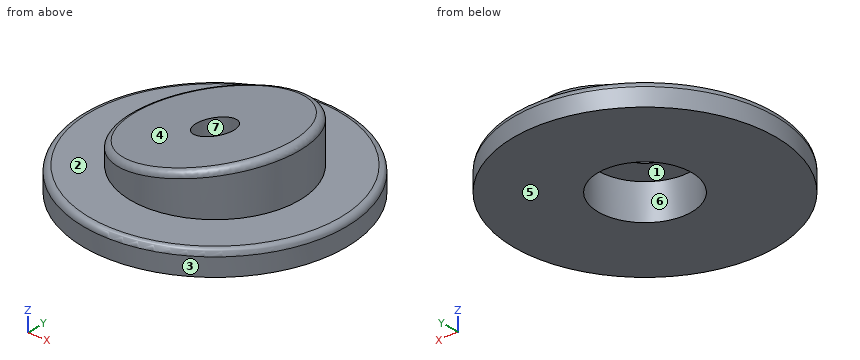
```python
from build123d import *

# Parameters (mm, degrees)
F0_R          = 11.1125
F0_R_2        = 7.14375
F1_DEPTH      = 2.032
F0_R_3        = 1.5875
F2_DEPTH      = 6.35
F4_DEPTH      = 11.1135
F4_DEPTH_BACK = 11.1135
F5_R          = 3.96875
F5_R_2        = 1.5875
F6_DEPTH      = 3.048
F7_R          = 0.508


with BuildPart() as f1:
    # F0 (on Top) → F1 (new body)
    with BuildSketch(Plane.XY):
        Circle(F0_R)
        Circle(F0_R_2, mode=Mode.SUBTRACT)
    extrude(amount=F1_DEPTH)

    # F0 (on Top) → F2 (join)
    with BuildSketch(Plane.XY):
        Circle(F0_R_2)
        Circle(F0_R_3, mode=Mode.SUBTRACT)
    extrude(amount=F2_DEPTH)

    # F3 (on Front) → F4 (cut, two sides)
    with BuildSketch(Plane.XZ) as f4_sk:
        Polygon((7.14375, 6.35), (-7.14375, 6.35), (-7.14375, 3.3864264842), align=None)
    extrude(amount=-F4_DEPTH, mode=Mode.SUBTRACT)
    extrude(f4_sk.sketch, amount=F4_DEPTH_BACK, mode=Mode.SUBTRACT)

    # F5 (on face) → F6 (cut)
    with BuildSketch(Plane(origin=(0, 0, 0), x_dir=(1, 0, 0), z_dir=(0, 0, -1))):
        Circle(F5_R)
        Circle(F5_R_2, mode=Mode.SUBTRACT)
    extrude(amount=-F6_DEPTH, mode=Mode.SUBTRACT)

    # F7
    f7_edges = [f1.edges().sort_by_distance(p)[0] for p in [
        (0, -7.14375, 4.868213),
        (0, 7.14375, 4.868213),
        (-11.1125, 0, 2.032),
    ]]
    fillet(f7_edges, radius=F7_R)


solid = f1.part
```
Source: CAD feature listing. Evaluate the final solid. Frame: model axes, mm. Face numbers are marked on the shaded views. A direction names the side the tool comes from. Coordinates: 2 decimals unless noted, no trailing zeros. Answer as a JSON object with one key per item and string values.
Q1. Draft query along X for the marked faces 4, 5, 6 and 7. Return one class per face: released by +X, released by -X, zero draft, split by the parting line, or undercut.
Ans:
{"face 4": "released by -X", "face 5": "zero draft", "face 6": "undercut", "face 7": "undercut"}
Q2. Material intervals for line 1 (Y direction, x = 0, z = 1.25); line 2 (Y direction, x = 0, z = 2.3); line 3 (Z direction, x = -7.75, y = 6.25), sorted ascending. Write a range as [from, to].
Ans:
{"line 1": "y = [-11.11, -3.97], [3.97, 11.11]", "line 2": "y = [-7.14, -3.97], [3.97, 7.14]", "line 3": "z = [0, 2.03]"}
Q3. First-contact query: pin 1 Ø5 at (x, y) = (0, 0) entering from +Z; pin 2 Ø1 at (x, y) = (8.5, 2.5) entering from +Z; pin 3 Ø2.5 at (x, y) = (-1, 0.5) entering from -Z. Flat tips, straight axial feed; report the tip coordinate or a pass-through.
Ans:
{"pin 1": "stops at z = 5.39", "pin 2": "stops at z = 2.03", "pin 3": "stops at z = 3.05"}
Q4. Set-up query: the marked faces 1, 2 and 3. Return all of +Z, -Z, +X, -X, +Y, -Y with unobstructed straight access to the full face (end or side cutting, diameter ignored); none if empty.
Ans:
{"face 1": "-Z", "face 2": "+Z", "face 3": "+Z, -Z"}
